from build123d import *

# Parameters (mm, degrees)
BOSS_EXTRUDE1_DEPTH = 64
SKETCH2_R           = 8.5
CUT_EXTRUDE1_DEPTH  = 109.081263889
SKETCH3_R           = 3
CUT_EXTRUDE2_DEPTH  = 113.967073095
SKETCH4_R           = 6
CUT_EXTRUDE3_DEPTH  = 3
CUT_EXTRUDE3_DRAFT  = -45


with BuildPart() as part:
    # Sketch1 → Boss-Extrude1 (new body)
    with BuildSketch(Plane.XY):
        with BuildLine():
            Line((-33.763886032, 52), (-72.003886032, 52))
            Line((-72.003886032, 52), (-72.003886032, 32))
            Line((-72.003886032, 32), (-36.003886032, 32))
            Line((-36.003886032, 32), (-36.003886032, 3))
            Line((-36.003886032, 3), (-31.863886032, 3))
            ThreePointArc((-31.863886032, 3), (0, 32.004800157), (31.863886032, 3))
            Line((31.863886032, 3), (36.003886032, 3))
            Line((36.003886032, 3), (36.003886032, 32))
            Line((36.003886032, 32), (72.003886032, 32))
            Line((72.003886032, 32), (72.003886032, 52))
            Line((72.003886032, 52), (33.763886032, 52))
            ThreePointArc((33.763886032, 52), (0, 62), (-33.763886032, 52))
        make_face()
    extrude(amount=BOSS_EXTRUDE1_DEPTH)

    # Sketch2 → Cut-Extrude1 (cut, through all)
    with BuildSketch(Plane(origin=(0, 52, 0), x_dir=(1, 0, 0), z_dir=(0, 1, 0))):
        with Locations(Location((-52.003886032, -32, 0), (0, 0, 180))):
            Circle(SKETCH2_R)
    cut_extrude1 = extrude(amount=-CUT_EXTRUDE1_DEPTH, mode=Mode.SUBTRACT)

    # Mirror1: Cut-Extrude1 across plane
    add(cut_extrude1.mirror(Plane(origin=(0, 0, 0), x_dir=(0, 0, 1), z_dir=(1, 0, 0))), mode=Mode.SUBTRACT)

    # Sketch3 → Cut-Extrude2 (cut, through all)
    with BuildSketch(Plane(origin=(0, 62, 0), x_dir=(1, 0, 0), z_dir=(0, 1, 0))):
        with Locations(Location((0, -32, 0), (0, 0, 270))):
            Circle(SKETCH3_R)
    extrude(amount=-CUT_EXTRUDE2_DEPTH, mode=Mode.SUBTRACT)


with BuildPart() as cut_extrude3_tool:
    # Sketch4 → Cut-Extrude3 (with draft: the straight prism first)
    with BuildSketch(Plane(origin=(0, 62, 0), x_dir=(1, 0, 0), z_dir=(0, 1, 0))):
        with Locations((0, -32)):
            Circle(SKETCH4_R)
    extrude(amount=-CUT_EXTRUDE3_DEPTH)
    # Cut-Extrude3: the draft: its side faces are tilted about the plane it starts from
    cut_extrude3_sides = [cut_extrude3_tool.faces().sort_by_distance(p)[0] for p in [
        (-6, 60.5, 32),
    ]]
    draft(cut_extrude3_sides, Plane(origin=(0, 62, 0), x_dir=(1, 0, 0), z_dir=(0, 1, 0)), CUT_EXTRUDE3_DRAFT)


with BuildPart() as part_1:
    add(part.part)

    # Cut-Extrude3: cut by cut_extrude3_tool
    add(cut_extrude3_tool.part, mode=Mode.SUBTRACT)


solid = part_1.part
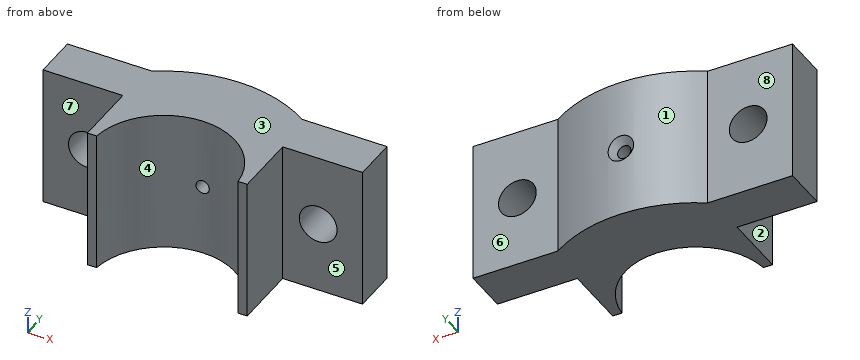
Source: CAD feature listing. Evaluate the final solid. Frame: model axes, mm. Face numbers are marked on the shaded views. A direction names the side the tool comes from. Round coordinates to 2 decimals unless told otherwise and drop trailing zeros. Loops run counter-clockwise (first coordinate to the right, second up) from the corner with the lowest first, then second, coordinate; pieces in that order, holes last. Notation, with made-up numbers: M 78.25,48 L 114.25,48 A18 cw 114.25,79 Z; hole C 40.25,82 d1. An arc over 180 degrees is marked long. Return JSON: item names as keys, results as strings. Group by question number.
1. Reachability of the marked faces 5, 6, 7 and 8 from +Z, -Z, +X, -X, +Y, -Y: full face, straight path, thin tool, end or side. Return the list, or none.
2. Section query D-D on z = 32. Output: boundary loops of the cut face in (x, y), and give its area (3 significant figures).
3. Section query A-A on y = 50. Output: boundary loops of the cut face in (x, z).
4. Mould query, pull axis X, two halves, no side actions, for the marked faces 1, 2, 3 and 4. Classes: released by +X, released by -X, zero draft, split by the parting line, or undercut.
5. Material intervals for line 1 along Z through (x, y) = (0, 52); line 2 along X through (y, z) = (14, 21.5); line 3 along Y through (x, z) = (-42, 57), sorted ascending. Write a range as from..to.
6. Section query B-B on z = 20. Output: boundary loops of the cut face in (x, y).
7. Pin query (flat end, axial travel): pin 1 (3 mm diameter, centred on x = -19.5, z = 50, fed in from -Y); pin 2 (9.5 mm diameter, centred on x = 0, z = 32, fed in from +Y); pin 3 (6 mm diameter, centred on x = 11, z = 49, fed in from -Y). Return the tip coordinate at first contact, or that it passes through.
8. Section query C-C on x = -47.5. Output: boundary loops of the cut face in (y, z), and give its area (3 significant figures).
Checks:
{
 "1": {"face 5": "+Z, -Z, +X, -Y", "face 6": "+Z, -Z, +X, +Y", "face 7": "+Z, -Z, -X, -Y", "face 8": "+Z, -Z, -X, +Y"},
 "2": {"outline": "M -72,32 L -60.5,32 L -60.5,52 L -72,52 Z; M -43.5,32 L -36,32 L -36,3 L -31.86,3 A32 cw -3,31.86 L -3,59 L -5.73,61.73 A62 ccw -33.76,52 L -43.5,52 Z; M 3,31.86 A32 cw 31.86,3 L 36,3 L 36,32 L 43.5,32 L 43.5,52 L 33.76,52 A62 ccw 5.73,61.73 L 3,59 Z; M 60.5,32 L 72,32 L 72,52 L 60.5,52 Z", "area": "3,140 mm²"},
 "3": {"outline": "M -72,0 L 72,0 L 72,64 L -72,64 Z; hole C -52,32 d17; hole C 0,32 d6; hole C 52,32 d17"},
 "4": {"face 1": "split by the parting line", "face 2": "released by -X", "face 3": "zero draft", "face 4": "undercut"},
 "5": {"line 1": "z = 0..29, 35..64", "line 2": "x = -36..-28.78, 28.78..36", "line 3": "y = 32..52"},
 "6": {"outline": "M -72,32 L -36,32 L -36,3 L -31.86,3 A32 cw 31.86,3 L 36,3 L 36,32 L 72,32 L 72,52 L 33.76,52 A62 ccw -33.76,52 L -72,52 Z"},
 "7": {"pin 1": "stops at y = 24.15", "pin 2": "stops at y = 60.75", "pin 3": "stops at y = 28.78"},
 "8": {"outline": "M 32,0 L 52,0 L 52,24.79 L 32,24.79 Z; M 32,39.21 L 52,39.21 L 52,64 L 32,64 Z", "area": "992 mm²"}
}
